from build123d import *

# Parameters (mm, degrees)
CYLINDER009_R     = 1.25
CYLINDER009_DEPTH = 20
CYLINDER010_R     = 1.25
CYLINDER010_DEPTH = 20
CYLINDER008_R     = 1.25
CYLINDER008_DEPTH = 20
CYLINDER011_R     = 1.25
CYLINDER011_DEPTH = 20
CYLINDER007_R     = 1.25
CYLINDER007_DEPTH = 20
CYLINDER006_R     = 1.25
CYLINDER006_DEPTH = 20
CYLINDER013_R     = 3
CYLINDER013_DEPTH = 3
CYLINDER017_R     = 3
CYLINDER017_DEPTH = 3
CYLINDER014_R     = 3
CYLINDER014_DEPTH = 3
CYLINDER015_R     = 3
CYLINDER015_DEPTH = 3
CYLINDER016_R     = 3
CYLINDER016_DEPTH = 3
CYLINDER012_R     = 3
CYLINDER012_DEPTH = 3
CYLINDER003_R     = 1.25
CYLINDER003_DEPTH = 7
CYLINDER005_R     = 1.25
CYLINDER005_DEPTH = 7
CYLINDER004_R     = 1.25
CYLINDER004_DEPTH = 7
CYLINDER002_R     = 1.25
CYLINDER002_DEPTH = 7
CYLINDER001_R     = 26
CYLINDER001_DEPTH = 13
CYLINDER_R        = 10
CYLINDER_DEPTH    = 20
BOX_W             = 70
BOX_H             = 70
BOX_DEPTH         = 20


with BuildPart() as zylinder009:
    # Cylinder009 → Cylinder009 (new body)
    with BuildSketch(Plane(origin=(-31, 31, 0), x_dir=(1, 0, 0), z_dir=(0, 0, 1))):
        Circle(CYLINDER009_R)
    extrude(amount=CYLINDER009_DEPTH)


with BuildPart() as zylinder010:
    # Cylinder010 → Cylinder010 (new body)
    with BuildSketch(Plane(origin=(-31, -31, 0), x_dir=(1, 0, 0), z_dir=(0, 0, 1))):
        Circle(CYLINDER010_R)
    extrude(amount=CYLINDER010_DEPTH)


with BuildPart() as zylinder008:
    # Cylinder008 → Cylinder008 (new body)
    with BuildSketch(Plane(origin=(31, -31, 0), x_dir=(1, 0, 0), z_dir=(0, 0, 1))):
        Circle(CYLINDER008_R)
    extrude(amount=CYLINDER008_DEPTH)


with BuildPart() as zylinder011:
    # Cylinder011 → Cylinder011 (new body)
    with BuildSketch(Plane(origin=(-31, 0, 0), x_dir=(1, 0, 0), z_dir=(0, 0, 1))):
        Circle(CYLINDER011_R)
    extrude(amount=CYLINDER011_DEPTH)


with BuildPart() as zylinder007:
    # Cylinder007 → Cylinder007 (new body)
    with BuildSketch(Plane(origin=(31, 0, 0), x_dir=(1, 0, 0), z_dir=(0, 0, 1))):
        Circle(CYLINDER007_R)
    extrude(amount=CYLINDER007_DEPTH)


with BuildPart() as fusion002:
    # Cylinder006 → Cylinder006 (new body)
    with BuildSketch(Plane(origin=(31, 31, 0), x_dir=(1, 0, 0), z_dir=(0, 0, 1))):
        Circle(CYLINDER006_R)
    extrude(amount=CYLINDER006_DEPTH)

    # Fusion002: union Zylinder009, Zylinder010, Zylinder008, Zylinder011, Zylinder007
    add(zylinder009.part)
    add(zylinder010.part)
    add(zylinder008.part)
    add(zylinder011.part)
    add(zylinder007.part)


with BuildPart() as zylinder013:
    # Cylinder013 → Cylinder013 (new body)
    with BuildSketch(Plane(origin=(-31, 31, 0), x_dir=(1, 0, 0), z_dir=(0, 0, 1))):
        Circle(CYLINDER013_R)
    extrude(amount=CYLINDER013_DEPTH)


with BuildPart() as zylinder017:
    # Cylinder017 → Cylinder017 (new body)
    with BuildSketch(Plane(origin=(-31, 0, 0), x_dir=(1, 0, 0), z_dir=(0, 0, 1))):
        Circle(CYLINDER017_R)
    extrude(amount=CYLINDER017_DEPTH)


with BuildPart() as zylinder014:
    # Cylinder014 → Cylinder014 (new body)
    with BuildSketch(Plane(origin=(-31, -31, 0), x_dir=(1, 0, 0), z_dir=(0, 0, 1))):
        Circle(CYLINDER014_R)
    extrude(amount=CYLINDER014_DEPTH)


with BuildPart() as zylinder015:
    # Cylinder015 → Cylinder015 (new body)
    with BuildSketch(Plane(origin=(31, -31, 0), x_dir=(1, 0, 0), z_dir=(0, 0, 1))):
        Circle(CYLINDER015_R)
    extrude(amount=CYLINDER015_DEPTH)


with BuildPart() as zylinder016:
    # Cylinder016 → Cylinder016 (new body)
    with BuildSketch(Plane(origin=(31, 0, 0), x_dir=(1, 0, 0), z_dir=(0, 0, 1))):
        Circle(CYLINDER016_R)
    extrude(amount=CYLINDER016_DEPTH)


with BuildPart() as fusion003:
    # Cylinder012 → Cylinder012 (new body)
    with BuildSketch(Plane(origin=(31, 31, 0), x_dir=(1, 0, 0), z_dir=(0, 0, 1))):
        Circle(CYLINDER012_R)
    extrude(amount=CYLINDER012_DEPTH)

    # Fusion001: union Zylinder013, Zylinder017, Zylinder014, Zylinder015, Zylinder016
    add(zylinder013.part)
    add(zylinder017.part)
    add(zylinder014.part)
    add(zylinder015.part)
    add(zylinder016.part)

    # Fusion003: union Fusion002
    add(fusion002.part)


with BuildPart() as zylinder003:
    # Cylinder003 → Cylinder003 (new body)
    with BuildSketch(Plane(origin=(-15, 0, 0), x_dir=(1, 0, 0), z_dir=(0, 0, 1))):
        Circle(CYLINDER003_R)
    extrude(amount=CYLINDER003_DEPTH)


with BuildPart() as zylinder005:
    # Cylinder005 → Cylinder005 (new body)
    with BuildSketch(Plane(origin=(0, -15, 0), x_dir=(1, 0, 0), z_dir=(0, 0, 1))):
        Circle(CYLINDER005_R)
    extrude(amount=CYLINDER005_DEPTH)


with BuildPart() as zylinder004:
    # Cylinder004 → Cylinder004 (new body)
    with BuildSketch(Plane(origin=(0, 15, 0), x_dir=(1, 0, 0), z_dir=(0, 0, 1))):
        Circle(CYLINDER004_R)
    extrude(amount=CYLINDER004_DEPTH)


with BuildPart() as fusion:
    # Cylinder002 → Cylinder002 (new body)
    with BuildSketch(Plane(origin=(15, 0, 0), x_dir=(1, 0, 0), z_dir=(0, 0, 1))):
        Circle(CYLINDER002_R)
    extrude(amount=CYLINDER002_DEPTH)

    # Fusion: union Zylinder003, Zylinder005, Zylinder004
    add(zylinder003.part)
    add(zylinder005.part)
    add(zylinder004.part)


with BuildPart() as zylinder001:
    # Cylinder001 → Cylinder001 (new body)
    with BuildSketch(Plane.XY.offset(7)):
        Circle(CYLINDER001_R)
    extrude(amount=CYLINDER001_DEPTH)


with BuildPart() as zylinder:
    # Cylinder → Cylinder (new body)
    with BuildSketch(Plane.XY):
        Circle(CYLINDER_R)
    extrude(amount=CYLINDER_DEPTH)


with BuildPart() as cut003:
    # Box → Box (new body)
    with BuildSketch(Plane(origin=(-35, -35, 0), x_dir=(1, 0, 0), z_dir=(0, 0, 1))):
        with Locations((35, 35)):
            Rectangle(BOX_W, BOX_H)
    extrude(amount=BOX_DEPTH)

    # Cut: cut Zylinder
    add(zylinder.part, mode=Mode.SUBTRACT)

    # Cut001: cut Zylinder001
    add(zylinder001.part, mode=Mode.SUBTRACT)

    # Cut002: cut Fusion
    add(fusion.part, mode=Mode.SUBTRACT)

    # Cut003: cut Fusion003
    add(fusion003.part, mode=Mode.SUBTRACT)


solid = cut003.part
Read the model definition and answer for the solid it produces. Units are mm, in the model's axes. A direction names the side the tool comes from. Round coordinates to 2 decimals unless told otherwise and drop trailing zeros. Write each loop counter-clockwise with the first axis right and the second up, starting at its lowest first coordinate (ties: lowest second). Pieces come first, ordered by that corner, then holes.
1. The part is cut by section B-B, the plane y = -31. Determine the outline of the cut face in (x, z).
2. Straight lines are drawn through the part: L1, parallel to Y at x = 0, z = 2.5; L2, parallel to Y at x = -31, z = 7.5; L3, parallel to X at y = 23.5, z = 15.5. For each, find the intervals that lie inside material, in ascending order.
3. The part is cut by section C-C, the plane z = 14.5. Determine the outline of the cut face in (x, y), then the cut area to 3 significant figures.
4. Which of the six approach directions +Z, -Z, +X, -X, +Y, -Y give full straight-line access (tool end or side, diameter ignored) to faces 1 (the face through (-34, 31, 1)), 2 (the face through (-20.633, -15.821, 13.409)), 3 (the face through (32.19, -30.62, 11.38))?
5. The part is cut by section A-A, the plane x = 0. Determine the outline of the cut face in (y, z).
6. The part is cut by section D-D, the plane y = -15. Determine the outline of the cut face in (x, z), then the cut area to 3 significant figures.
7. Given pin 1 Ø2 at (x, y) = (0, 15) entering from +Z; pin 2 Ø4 at (x, y) = (15, 0) entering from +Z, each flat-ended and moving along its own axis, determine where each tip first touches the part or whether it passes through.
Values:
1. outline: (-35, 0) - (-34, 0) - (-34, 3) - (-32.25, 3) - (-32.25, 20) - (-35, 20) - close; (-29.75, 3) - (-28, 3) - (-28, 0) - (28, 0) - (28, 3) - (29.75, 3) - (29.75, 20) - (-29.75, 20) - close; (32.25, 3) - (34, 3) - (34, 0) - (35, 0) - (35, 20) - (32.25, 20) - close
2. L1: y = -35 to -16.25, -13.75 to -10, 10 to 13.75, 16.25 to 35
2. L2: y = -35 to -32.25, -29.75 to -1.25, 1.25 to 29.75, 32.25 to 35
2. L3: x = -35 to -11.12, 11.12 to 35
3. outline: (-35, -35) - (35, -35) - (35, 35) - (-35, 35) - close; hole circle Ø2.5 at (-31, -31); hole circle Ø2.5 at (-31, 0); hole circle Ø2.5 at (-31, 31); hole circle Ø52 at (0, 0); hole circle Ø2.5 at (31, -31); hole circle Ø2.5 at (31, 0); hole circle Ø2.5 at (31, 31)
3. area: 2,750 mm2
4. face 1: -Z
4. face 2: +Z
4. face 3: +Z, -Z
5. outline: (-35, 0) - (-16.25, 0) - (-16.25, 7) - (-26, 7) - (-26, 20) - (-35, 20) - close; (-13.75, 0) - (-10, 0) - (-10, 7) - (-13.75, 7) - close; (10, 0) - (13.75, 0) - (13.75, 7) - (10, 7) - close; (16.25, 0) - (35, 0) - (35, 20) - (26, 20) - (26, 7) - (16.25, 7) - close
6. outline: (-35, 0) - (-1.25, 0) - (-1.25, 7) - (-21.24, 7) - (-21.24, 20) - (-35, 20) - close; (1.25, 0) - (35, 0) - (35, 20) - (21.24, 20) - (21.24, 7) - (1.25, 7) - close
6. area: 830 mm2
7. pin 1: passes through
7. pin 2: stops at z = 7
